Design review of the part shown in the three views and the two pictorial views. Dimensions are in mm from the part's minimum x, y and z. Give positions to 0.01 mm unless a question says otherwise; leave off trailing zeros. Order: outer loops, then holes, each group sorted by start corner. A loop starts at its lowest first (then second) coordinate and runs counter-clockwise, first axis right, second up. Notation, with made-up numbers: M 14,19 L 40,19 A15 cw 40,43 Z; hole C 51,65.5 d2. An arc over 180 degrees is marked long. Answer as a JSON object with one key per item and string values.
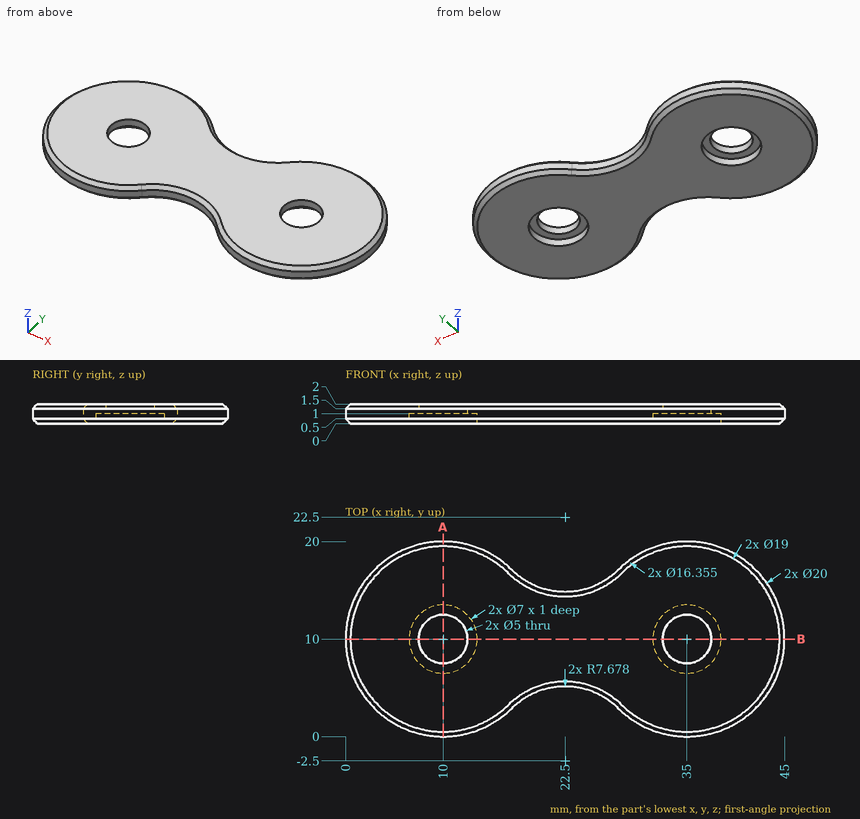
(1) We need section A-A (x = 10). Write out the cut boundary in (y, z), plus the area to 3 significant figures.
Checked values:
{"outline": "M 0,0.5 L 0.5,0 L 6.5,0 L 6.5,1 L 7.5,1 L 7.5,2 L 0.5,2 L 0,1.5 Z; M 12.5,1 L 13.5,1 L 13.5,0 L 19.5,0 L 20,0.5 L 20,1.5 L 19.5,2 L 12.5,2 Z", "area": "27.5 mm^2"}
(2) Insertion check: pin 1 (3 mm diameter, centred on x = 35, y = 10, fed in from +Z); pin 2 (1 mm diameter, centred on y = 15, z = 1, fed in from -X). Each pin has a flat end and moves straight along its axis. Give the tip position at first contact, or say it passes through.
Checked values:
{"pin 1": "passes through", "pin 2": "stops at x = 1.07"}
(3) We need section B-B (y = 10). Write out the cut boundary in (x, z).
Checked values:
{"outline": "M 0,0.5 L 0.5,0 L 6.5,0 L 6.5,1 L 7.5,1 L 7.5,2 L 0.5,2 L 0,1.5 Z; M 12.5,1 L 13.5,1 L 13.5,0 L 31.5,0 L 31.5,1 L 32.5,1 L 32.5,2 L 12.5,2 Z; M 37.5,1 L 38.5,1 L 38.5,0 L 44.5,0 L 45,0.5 L 45,1.5 L 44.5,2 L 37.5,2 Z"}
(4) To check wall thickness, follow L1, parallel to X at y = 8.5, z = 1.05; L2, parallel to Y at x = 10, z = 1.4; L3, parallel to X at y = 11.5, z = 1.7 (1 decimal). State the ranges of each line that lie inside material, in increasing order. Write a range as from..to.
Checked values:
{"L1": "x = 0.11..8, 12..33, 37..44.89", "L2": "y = 0..7.5, 12.5..20", "L3": "x = 0.3..8, 12..33, 37..44.7"}
